```python
from build123d import *

# Parameters (mm, degrees)
F1_DEPTH = 8.001


with BuildPart() as f1:
    # F0 (on Front) → F1 (new body)
    with BuildSketch(Plane.XZ):
        with BuildLine():
            Line((-25.4, 0), (0, 0))
            Line((0, 0), (0, 44.122111))
            ThreePointArc((0, 44.122111), (-3.183424, 51.807576), (-10.868889, 54.991))
            Line((-10.868889, 54.991), (-14.531116, 54.991))
            ThreePointArc((-14.531116, 54.991), (-22.216577, 51.807577), (-25.4, 44.122116))
            Line((-25.4, 44.122116), (-25.4, 0))
        make_face()
    extrude(amount=F1_DEPTH)


solid = f1.part
```
Here's how the part is built. I have some questions about the finished solid (model axes, mm). Give positions to 0.01 mm unless a question says otherwise; leave off trailing zeros. Loops run counter-clockwise (first coordinate to the right, second up) from the corner with the lowest first, then second, coordinate; pieces in that order, holes last. Notation, with made-up numbers: M 49,-30.5 L 68,-30.5 A16 ccw 68,-22.5 Z; hole C 25,70 d6. An arc over 180 degrees is marked long. Return JSON: item names as keys, results as strings.
Item 1: I'm going to push a flat-ended pin straight in: pin 1 Ø1 at (y, z) = (-4.5, 47.5) entering from -X. Where does the tip first touch, or does it pass through?
A:
{"pin 1": "stops at x = -25.01"}
Item 2: Imagine slicing it at A-A on y = -4. List the corners of the cut face in (x, z) for me, then the cut area to 3 significant figures.
A:
{"outline": "M -25.4,0 L 0,0 L 0,44.12 A10.87 ccw -10.87,54.99 L -14.53,54.99 A10.87 ccw -25.4,44.12 Z", "area": "1,350 mm^2"}
Item 3: Please list where these lines run through material, in increasing order: line 1 (Z direction, x = -22, y = -1.5); line 2 (Z direction, x = -8.5, y = -7.5); line 3 (X direction, y = -2.25, z = 51.5).
A:
{"line 1": "z = 0 to 52.02", "line 2": "z = 0 to 54.73", "line 3": "x = -22.51 to -2.89"}
Item 4: Imagine slicing it at B-B on z = 50.5. List the corners of the cut face in (x, y) for me.
A:
{"outline": "M -23.33,-8 L -2.07,-8 L -2.07,0 L -23.33,0 Z"}
Item 5: Imagine slicing it at C-C on x = -1.25. List the corners of the cut face in (y, z) for me, then the cut area to 3 significant figures.
A:
{"outline": "M -8,0 L 0,0 L 0,49.18 L -8,49.18 Z", "area": "394 mm^2"}
